Geometry: final body of the model. Coordinates: model frame, mm. Give positions to 0.01 mm unless a question says otherwise; leave off trailing zeros. Write each loop counter-clockwise with the first axis right and the second up, starting at its lowest first coordinate (ties: lowest second). Pieces come first, ordered by that corner, then holes.
from build123d import *

# Parameters (mm, degrees)
SKETCH1_R           = 1.5
SKETCH1_R_2         = 1.4
BOSS_EXTRUDE1_DEPTH = 3.18
CUT_EXTRUDE1_DEPTH  = 10


with BuildPart() as part:
    # Sketch1 → Boss-Extrude1 (new body)
    with BuildSketch(Plane.XY):
        Polygon((-201.59, 50), (-201.59, 12.5), (-198.41, 12.5), (-198.41, 1.5), (-194.41, 1.5), (-194.41, 4.5), (-191.41, 4.5), (-191.41, 1.5), (-188.59, 1.5), (-188.59, -1.5), (-191.41, -1.5), (-191.41, -4.5), (-194.41, -4.5), (-194.41, -1.5), (-198.41, -1.5), (-198.41, -12.5), (-201.59, -12.5), (-201.59, -50), (-10.91, -50), (-10.91, -53.18), (14.09, -53.18), (14.09, -50), (201.59, -50), (201.59, -12.5), (210.59, -12.5), (210.59, 12.5), (201.59, 12.5), (201.59, 50), (14.09, 50), (14.09, 53.18), (-10.91, 53.18), (-10.91, 50), align=None)
        with Locations(Location((1.59, 51.59, 0), (0, 0, 180))):
            Circle(SKETCH1_R, mode=Mode.SUBTRACT)
        with Locations(Location((1.59, -51.59, 0), (0, 0, 180))):
            Circle(SKETCH1_R, mode=Mode.SUBTRACT)
        with Locations(Location((208.39, 8, 0), (0, 0, 180))):
            Circle(SKETCH1_R_2, mode=Mode.SUBTRACT)
        with Locations(Location((208.39, -8, 0), (0, 0, 180))):
            Circle(SKETCH1_R_2, mode=Mode.SUBTRACT)
    extrude(amount=BOSS_EXTRUDE1_DEPTH)

    # Sketch2 → Cut-Extrude1 (cut)
    with BuildSketch(Plane.XY.offset(3.18)):
        Polygon((-173.347543098, 4.310263234), (152.804450916, 4.310263234), (201.59, 4.310263234), (212.087554944, 4.310263234), (212.087554944, -4.889736766), (201.37, -4.889736766), (196.652456902, -4.889736766), (-173.347543098, -4.889736766), align=None)
    extrude(amount=-CUT_EXTRUDE1_DEPTH, mode=Mode.SUBTRACT)


solid = part.part
Q1. Ray query, line 1 along Y through (x, z) = (208.39, 1.6); line 2 along X through (y, z) = (8, 1.3); line 3 along Y through (x, z) = (157.5, 2.35). Return the intervals inside material, ascending.
Filled sheet:
line 1: y = -12.5 to -9.4, -6.6 to -4.89, 4.31 to 6.6, 9.4 to 12.5
line 2: x = -198.41 to 206.99, 209.79 to 210.59
line 3: y = -50 to -4.89, 4.31 to 50
Q2. Section B-B on z = 1.55. Count the separate pieces of the cut face and the enclosed holes in it, plus the area to 3 significant figures.
Filled sheet:
separate pieces: 1
enclosed holes: 4
area: 37,000 mm2
Q3. Pin query (flat end, axial travel): P1, Ø12, axis at x = -129.5, y = 3.5, coming from the -Z side; P2, Ø1, axis at y = 1.5, z = 1.5, coming from the -X side; P3, Ø1.6, axis at x = 131, z = 1.5, coming from the +Y side; P4, Ø1.5, axis at y = -3.5, z = 2, coming from the +X side. Return the tip coordinate at first contact, or that it passes through.
Filled sheet:
P1: stops at z = 0
P2: stops at x = -198.41
P3: stops at y = 50
P4: stops at x = -173.35
Q4. Section C-C on y = 35. Output: boundary loops of the cut face in (x, z), plus the area to 3 significant figures.
Filled sheet:
outline: (-201.59, 0) - (201.59, 0) - (201.59, 3.18) - (-201.59, 3.18) - close
area: 1,280 mm2
Q5. Section A-A on x = -115. Output: boundary loops of the cut face in (y, z).
Filled sheet:
outline: (-50, 0) - (-4.89, 0) - (-4.89, 3.18) - (-50, 3.18) - close; (4.31, 0) - (50, 0) - (50, 3.18) - (4.31, 3.18) - close
